from build123d import *

# Parameters (mm, degrees)
STOCK_U_HANDLE_1_START     = -1.5
STOCK_U_HANDLE_1_OUTLINE_R = 1.2
STOCK_U_HANDLE_1_DEPTH     = 3
FILLET1_R                  = 0.5


# Read off the part's stored shape, not the designer's step: Stock-u-handle-1
with BuildPart() as part:
    # Stock-u-handle-1 outline → Stock-u-handle-1 (new body)
    with BuildSketch(Plane(origin=(0, 0, 0), x_dir=(1, 0, 0), z_dir=(0, 1, 0)).offset(STOCK_U_HANDLE_1_START)):
        with BuildLine():
            Line((5, -32.5), (-5, -32.5))
            Line((-5, -32.5), (-5, -37.5))
            ThreePointArc((-5, -37.5), (0, -42.5), (5, -37.5))
            Line((5, -37.5), (5, -32.5))
        make_face()
        with Locations((1.590990258, -38.590990258)):
            Circle(STOCK_U_HANDLE_1_OUTLINE_R, mode=Mode.SUBTRACT)
        with Locations((-1.590990258, -35.409009742)):
            Circle(STOCK_U_HANDLE_1_OUTLINE_R, mode=Mode.SUBTRACT)
    extrude(amount=STOCK_U_HANDLE_1_DEPTH)

    # Fillet1
    fillet1_edges = [part.edges().sort_by_distance(p)[0] for p in [
        (-5, 0, 32.5),
        (5, 0, 32.5),
    ]]
    fillet(fillet1_edges, radius=FILLET1_R)


solid = part.part
Model file for the job. Use its own axes, mm. Give positions to 0.01 mm unless a question says otherwise; leave off trailing zeros. Loops run counter-clockwise (first coordinate to the right, second up) from the corner with the lowest first, then second, coordinate; pieces in that order, holes last. Notation, with made-up numbers: (-8, 82) -> (49, 82) arc R30 cw to (49, 120) -> close; hole circle Ø3 at (-39.75, 87.5). An arc over 180 degrees is marked (long way). Use a Markdown table: item, result. Add a question column.
(1) Mould opens along X. For faces 1 (the flat face through (0, -1.5, 37)), 2 (the flat face through (5, 0, 35)), 3 (the cylindrical face through (1.43, -0.02, 37.4)) say: +X half, -X half, draft (parallel to the pull), parting line (faces both ways), or undercut.
(2) Wall check: line 1 along X through (y, z) = (-0.25, 34.5); line 2 along X through (y, z) = (-0.45, 35.5); line 3 along Z through (x, y) = (-0.75, 0.35) (3 decimals). Give the ranges that are in metal, low to high.
(3) Drop flat-ended pins along their axis: pin 1 Ø2 at (x, z) = (1.59, 38.59) entering from -Y; pin 2 Ø1.5 at (y, z) = (0.5, 41.5) entering from -X. Give the stop position or say it passes through.
(4) Slice it at B-B on y = 0.1. List the corners of the cut face in (x, z).
(5) Slice it at C-C on z = 40.5. List the corners of the cut face in (x, y), and give its area (3 significant figures).
(6) Slice it at A-A on x = 1.75. List the corners of the cut face in (y, z), and give its area (3 significant figures).
(7) Slice it at D-D on x = -2.5. List the corners of the cut face in (y, z), and give its area (3 significant figures).
Filled sheet:
| question | item | result |
|---|---|---|
| 1 | face 1 | draft |
| 1 | face 2 | +X half |
| 1 | face 3 | undercut |
| 2 | line 1 | -5 to -2.37, -0.81 to 5 |
| 2 | line 2 | -5 to -2.79, -0.39 to 5 |
| 2 | line 3 | 32.5 to 34.553, 36.265 to 42.443 |
| 3 | pin 1 | through |
| 3 | pin 2 | x = -3.8 |
| 4 | outline | (-5, 33) arc R0.5 ccw to (-4.5, 32.5) -> (4.5, 32.5) arc R0.5 ccw to (5, 33) -> (5, 37.5) arc R5 ccw to (-5, 37.5) -> close; hole circle Ø2.4 at (-1.59, 35.41); hole circle Ø2.4 at (1.59, 38.59) |
| 5 | outline | (-4, -1.5) -> (4, -1.5) -> (4, 1.5) -> (-4, 1.5) -> close |
| 5 | area | 24.0 mm2 |
| 6 | outline | (-1.5, 32.5) -> (1.5, 32.5) -> (1.5, 37.4) -> (-1.5, 37.4) -> close; (-1.5, 39.78) -> (1.5, 39.78) -> (1.5, 42.18) -> (-1.5, 42.18) -> close |
| 6 | area | 21.9 mm2 |
| 7 | outline | (-1.5, 32.5) -> (1.5, 32.5) -> (1.5, 34.63) -> (-1.5, 34.63) -> close; (-1.5, 36.19) -> (1.5, 36.19) -> (1.5, 41.83) -> (-1.5, 41.83) -> close |
| 7 | area | 23.3 mm2 |
